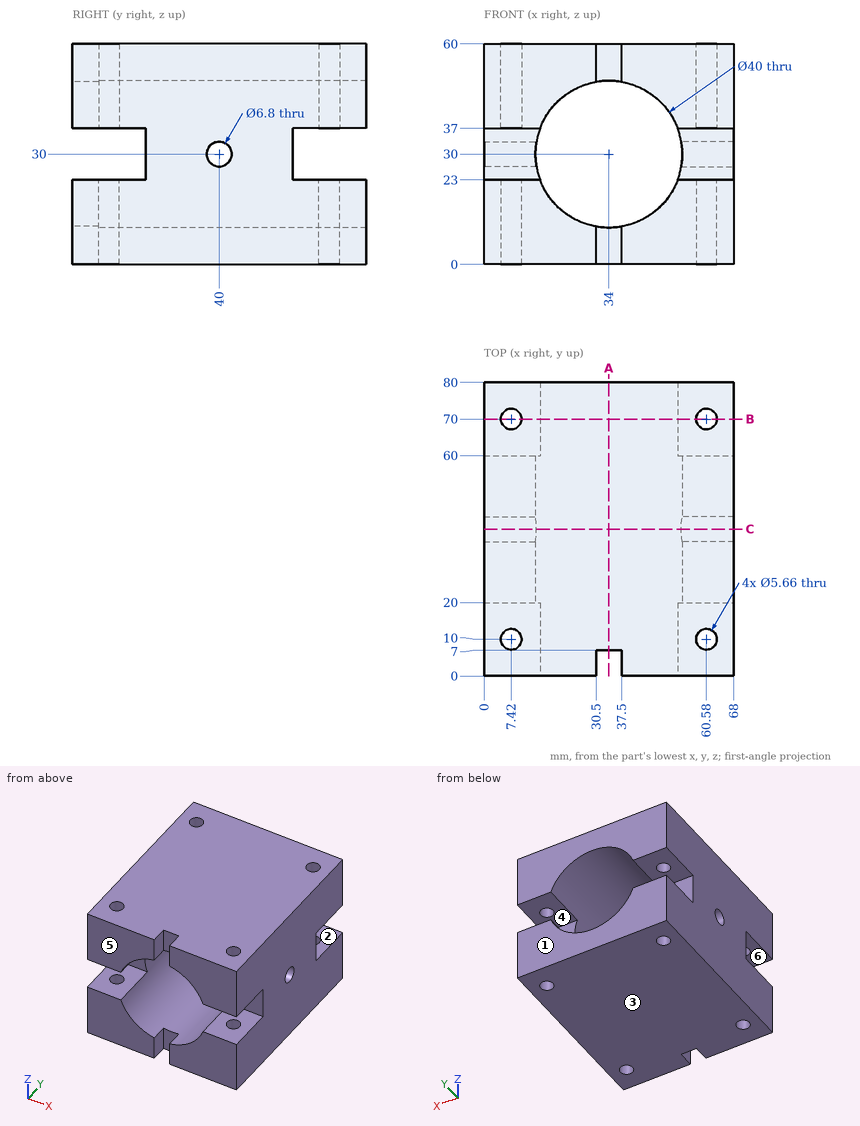
Part print with two shaded views. Sizes in mm from the minimum x, y, z corner. A direction names the side the tool comes from. Round coordinates to 2 decimals unless told otherwise and drop trailing zeros. Loops run counter-clockwise (first coordinate to the right, second up) from the corner with the lowest first, then second, coordinate; pieces in that order, holes last.
Item 1: Which spindle directions (+Z, -Z, +X, -X, +Y, -Y) get a long thin tool onto all of the face, cutting with end or side? Do the marked faces 4, 5 and 6. Say none if no direction does.
Item 2: Drill centre lines: line 1 along Y through (x, z) = (60.58, 9.5); line 2 along Z through (x, y) = (33.5, 26.5); line 3 along Y through (x, z) = (60.5, 30). Where is each one in solid material? Low to high.
Item 3: Saw through at A-A (x = 34). List the corners of the cut face in (y, z), then the cut area to 3 significant figures.
Item 4: Two-plate mould, pull along Z, no slides. Class the marked faces 1, 2 and 3: released by +Z, released by -Z, zero draft, split by the parting line, or undercut.
Item 5: Saw through at B-B (y = 70). State how many separate pieces and enclosed holes the cut face has, then the cut area to 3 significant figures.
Item 6: Pin check, flat tip, straight feed: P1, Ø3.5, axis at x = 60.58, y = 10, coming from the +Z side. Stop position of the tip, or through.
Item 7: Saw through at C-C (y = 40). List the corners of the cut face in (x, z), then the cut area to 3 significant figures.
Worked answers:
1. face 4: +X, -X, +Y
1. face 5: +Z, -Z, +X, -X, -Y
1. face 6: +X, -X, -Y
2. line 1: y = 0 to 7.17, 12.83 to 67.17, 72.83 to 80
2. line 2: z = 0 to 10.01, 49.99 to 60
2. line 3: y = 20 to 36.6, 43.4 to 60
3. outline: (7, 0) - (80, 0) - (80, 10) - (7, 10) - close; (7, 50) - (80, 50) - (80, 60) - (7, 60) - close
3. area: 1,460 mm2
4. face 1: zero draft
4. face 2: undercut
4. face 3: released by -Z
5. separate pieces: 6
5. enclosed holes: 0
5. area: 1,900 mm2
6. P1: passes through
7. outline: (0, 0) - (68, 0) - (68, 26.6) - (53.71, 26.6) arc R20 cw to (14.29, 26.6) - (0, 26.6) - close; (0, 33.4) - (14.29, 33.4) arc R20 cw to (53.71, 33.4) - (68, 33.4) - (68, 60) - (0, 60) - close
7. area: 2,630 mm2
